from build123d import *

# Parameters (mm, degrees)
EXTRUDE_1_DEPTH        = 32.5
HOLE_WIZARD_M6_1_D     = 5
HOLE_WIZARD_M6_1_DEPTH = 10
HOLE_WIZARD_M6_1_TIP   = 1.502151548


with BuildPart() as part:
    # 草图1 → 凸台-拉伸1 (new body, symmetric)
    with BuildSketch(Plane.XY):
        with BuildLine():
            Line((-17.5, 0), (-7.5, 10))
            ThreePointArc((-7.5, 10), (0, 32.5), (7.5, 10))
            Line((7.5, 10), (17.5, 0))
            Line((17.5, 0), (30, 0))
            Line((30, 0), (30, 47))
            Line((30, 47), (-30, 47))
            Line((-30, 47), (-30, 0))
            Line((-30, 0), (-17.5, 0))
        make_face()
    extrude(amount=EXTRUDE_1_DEPTH, both=True)

    # M6 螺纹孔1
    with Locations(Plane(origin=(-20, 47, -20), x_dir=(1, 0, 0), z_dir=(0, 1, 0))):
        with Locations((0, 0), (40, 0), (40, -40), (0, -40)):
            Hole(HOLE_WIZARD_M6_1_D / 2, depth=HOLE_WIZARD_M6_1_DEPTH)
            with Locations((0, 0, -(HOLE_WIZARD_M6_1_DEPTH + HOLE_WIZARD_M6_1_TIP / 2))):  # 118° drill point
                Cone(0, HOLE_WIZARD_M6_1_D / 2, HOLE_WIZARD_M6_1_TIP, mode=Mode.SUBTRACT)


solid = part.part
Build history of the part. All positions in model axes, mm. A direction names the side the tool comes from. Give positions to 0.01 mm unless a question says otherwise; leave off trailing zeros. Write each loop counter-clockwise with the first axis right and the second up, starting at its lowest first coordinate (ties: lowest second). Pieces come first, ordered by that corner, then holes. Notation, with made-up numbers: (60.25, -12) - (83.25, -12) arc R21 cw to (83.25, 6) - close; hole circle Ø8 at (9.25, 2). An arc over 180 degrees is marked (long way). Use one line per item in the form item = value. Start each with the question number.
1. Band-saw the part on D-D on x = 0. Write the cut outline in (y, z).
2. Drop flat-ended pins along their axis: pin 1 Ø1.5 at (x, z) = (7.5, -6.5) entering from -Y; pin 2 Ø4 at (x, z) = (-20, 20) entering from +Y; pin 3 Ø3 at (x, z) = (20, 20) entering from -Y; pin 4 Ø1 at (x, z) = (14, -22.5) entering from -Y. Give the stop position or say it passes through.
3. 3-axis set-ups, long thin cutter, end or side, ignore diameter. For faces 4 (the face through (-0.437, 32.492, 0.455)), 5 (the face through (21.84, 41.93, -21.69)), 6 (the face through (-12.6, 4.9, 0.5)): which of +Z, -Z, +X, -X, +Y, -Y reach the whole face in a straight line?
4. Probe line 1 (Z direction, x = 20, y = 43); line 2 (X direction, y = 43.25, z = -20); line 3 (X direction, y = 43, z = -18.5). List the from-to ranges inside material, lowest first. Write a range as [from, to].
5. Two-plate mould, pull along X, no slides. Class faces 1 (the face through (12.4, 5.1, 0.5)), 2 (the face through (0, 34, -32.5)), 3 (the face through (30, 23, 0)): released by +X, released by -X, zero draft, split by the parting line, or undercut.
6. Band-saw the part on C-C on x = -10.5. Write the cut outline in (y, z), plus the area to 3 significant figures.
7. Band-saw the part on B-B on z = -13.5. Write the cut outline in (x, y), plus the area to 3 significant figures.
8. Band-saw the part on A-A on y = 7.5. Write the cut outline in (x, z).
Conclusion:
q1.outline = (32.5, -32.5) - (47, -32.5) - (47, 32.5) - (32.5, 32.5) - close
q2.pin_1 = 9.25
q2.pin_2 = 36.7
q2.pin_3 = 0
q2.pin_4 = 3
q3.face_4 = +Z, -Z
q3.face_5 = +Y
q3.face_6 = +Z, -Z, -Y
q4.line_1 = [-32.5, -22.5], [-17.5, 17.5], [22.5, 32.5]
q4.line_2 = [-30, -22.5], [-17.5, 17.5], [22.5, 30]
q4.line_3 = [-30, -22], [-18, 18], [22, 30]
q5.face_1 = undercut
q5.face_2 = zero draft
q5.face_3 = released by +X
q6.outline = (7, -32.5) - (13.22, -32.5) - (13.22, 32.5) - (7, 32.5) - close; (26.78, -32.5) - (47, -32.5) - (47, 32.5) - (26.78, 32.5) - close
q6.area = 1,720 mm²
q7.outline = (-30, 0) - (-17.5, 0) - (-7.5, 10) arc R12.5 cw (long way) to (7.5, 10) - (17.5, 0) - (30, 0) - (30, 47) - (-30, 47) - close
q7.area = 2,100 mm²
q8.outline = (-30, -32.5) - (-10, -32.5) - (-10, 32.5) - (-30, 32.5) - close; (10, -32.5) - (30, -32.5) - (30, 32.5) - (10, 32.5) - close
